```python
from build123d import *

# Parameters (mm, degrees)
SKETCH_1_W          = 35.997280892
SKETCH_1_H          = 36.282611102
SKETCH_1_W_2        = 35
SKETCH_1_H_2        = 32
EXTRUDE_1_DEPTH     = 65
SKETCH_1_3_W        = 35.997280892
SKETCH_1_3_H        = 36.282611102
SKETCH_1_3_W_2      = 35
SKETCH_1_3_H_2      = 32
EXTRUDE_2_DEPTH     = 2
SKETCH_2_R          = 1
CUT_EXTRUDE_1_DEPTH = 74.759079051
SKETCH_3_R          = 2
CUT_EXTRUDE_2_DEPTH = 1
EXTRUDE_3_DEPTH     = 4.5
EXTRUDE_4_DEPTH     = 30


with BuildPart() as part:
    # Sketch 1 → Extrude 1 (new body)
    # profile 1 of 5: a face of its own
    with BuildSketch(Plane(origin=(0, 0, 0), x_dir=(1, 0, 0), z_dir=(0, 1, 0))):
        Polygon((-14.328756252, 21.811189745), (14.328756252, 21.811189745), (17.998640446, 18.141305551), (-17.998640446, 18.141305551), align=None)
    # profile 2 of 5: a face of its own
    with BuildSketch(Plane(origin=(0, 0, 0), x_dir=(1, 0, 0), z_dir=(0, 1, 0))):
        Rectangle(SKETCH_1_W, SKETCH_1_H)
        Rectangle(SKETCH_1_W_2, SKETCH_1_H_2, mode=Mode.SUBTRACT)
    # profile 3 of 5: a face of its own
    with BuildSketch(Plane(origin=(0, 0, 0), x_dir=(1, 0, 0), z_dir=(0, 1, 0))):
        Polygon((-21.809945997, -14.33), (-21.809945997, 14.33), (-17.998640446, 18.141305551), (-17.998640446, -18.141305551), align=None)
    # profile 4 of 5: a face of its own
    with BuildSketch(Plane(origin=(0, 0, 0), x_dir=(1, 0, 0), z_dir=(0, 1, 0))):
        Polygon((14.328756252, -21.811189745), (-14.328756252, -21.811189745), (-17.998640446, -18.141305551), (17.998640446, -18.141305551), align=None)
    # profile 5 of 5: a face of its own
    with BuildSketch(Plane(origin=(0, 0, 0), x_dir=(1, 0, 0), z_dir=(0, 1, 0))):
        Polygon((21.809945997, 14.33), (21.809945997, -14.33), (17.998640446, -18.141305551), (17.998640446, 18.141305551), align=None)
    extrude(amount=EXTRUDE_1_DEPTH)

    # Sketch 1_3 → Extrude 2 (add)
    # profile 1 of 6: a face of its own
    with BuildSketch(Plane(origin=(0, 0, 0), x_dir=(1, 0, 0), z_dir=(0, 1, 0))):
        Polygon((-21.809945997, -14.33), (-21.809945997, 14.33), (-17.998640446, 18.141305551), (-17.998640446, -18.141305551), align=None)
    # profile 2 of 6: a face of its own
    with BuildSketch(Plane(origin=(0, 0, 0), x_dir=(1, 0, 0), z_dir=(0, 1, 0))):
        Rectangle(SKETCH_1_3_W, SKETCH_1_3_H)
        Rectangle(SKETCH_1_3_W_2, SKETCH_1_3_H_2, mode=Mode.SUBTRACT)
    # profile 3 of 6: a face of its own
    with BuildSketch(Plane(origin=(0, 0, 0), x_dir=(1, 0, 0), z_dir=(0, 1, 0))):
        Rectangle(SKETCH_1_3_W_2, SKETCH_1_3_H_2)
    # profile 4 of 6: a face of its own
    with BuildSketch(Plane(origin=(0, 0, 0), x_dir=(1, 0, 0), z_dir=(0, 1, 0))):
        Polygon((-14.328756252, 21.811189745), (14.328756252, 21.811189745), (17.998640446, 18.141305551), (-17.998640446, 18.141305551), align=None)
    # profile 5 of 6: a face of its own
    with BuildSketch(Plane(origin=(0, 0, 0), x_dir=(1, 0, 0), z_dir=(0, 1, 0))):
        Polygon((21.809945997, 14.33), (21.809945997, -14.33), (17.998640446, -18.141305551), (17.998640446, 18.141305551), align=None)
    # profile 6 of 6: a face of its own
    with BuildSketch(Plane(origin=(0, 0, 0), x_dir=(1, 0, 0), z_dir=(0, 1, 0))):
        Polygon((14.328756252, -21.811189745), (-14.328756252, -21.811189745), (-17.998640446, -18.141305551), (17.998640446, -18.141305551), align=None)
    extrude(amount=-EXTRUDE_2_DEPTH)

    # Sketch 2 → Cut-Extrude 1 (cut, through all)
    with BuildSketch(Plane.XZ.offset(2)):
        with Locations(Location((-3.809945997, 8, 0), (0, 0, 270))):
            Circle(SKETCH_2_R)
        with Locations(Location((-3.809945997, -8, 0), (0, 0, 270))):
            Circle(SKETCH_2_R)
    extrude(amount=-CUT_EXTRUDE_1_DEPTH, mode=Mode.SUBTRACT)

    # Sketch 3 → Cut-Extrude 2 (cut)
    with BuildSketch(Plane(origin=(0, 0, 0), x_dir=(1, 0, 0), z_dir=(0, 1, 0))):
        with Locations(Location((-3.809945997, 8, 0), (0, 0, 270))):
            Circle(SKETCH_3_R)
        with Locations(Location((-3.809945997, -8, 0), (0, 0, 270))):
            Circle(SKETCH_3_R)
    extrude(amount=-CUT_EXTRUDE_2_DEPTH, mode=Mode.SUBTRACT)

    # Sketch 4 → Extrude 3 (add)
    with BuildSketch(Plane.XZ.offset(2)):
        Polygon((-14.328756252, 21.811189745), (-19.27850372, 16.861442277), (-17.864290158, 15.447228714), (-12.91454269, 20.396976183), align=None)
        Polygon((19.27850372, 16.861442277), (14.328756252, 21.811189745), (12.91454269, 20.396976183), (17.864290158, 15.447228714), align=None)
        Polygon((12.91454269, -20.396976183), (14.328756252, -21.811189745), (19.27850372, -16.861442277), (17.864290158, -15.447228714), align=None)
        Polygon((-17.864290158, -15.447228714), (-19.27850372, -16.861442277), (-14.328756252, -21.811189745), (-12.91454269, -20.396976183), align=None)
    extrude(amount=EXTRUDE_3_DEPTH)

    # Sketch 5 → Extrude 4 (add)
    with BuildSketch(Plane.XZ.offset(2)):
        with BuildLine():
            ThreePointArc((8.828756252, 21.811189745), (5.891921221, 22.764586231), (4.075073469, 25.261189745))
            Line((4.075073469, 25.261189745), (4.075073469, 21.811189745))
            Line((4.075073469, 21.811189745), (8.828756252, 21.811189745))
        make_face()
        with BuildLine():
            ThreePointArc((13.582439035, 25.261189745), (11.765591283, 22.764586231), (8.828756252, 21.811189745))
            Line((8.828756252, 21.811189745), (13.582439035, 21.811189745))
            Line((13.582439035, 21.811189745), (13.582439035, 25.261189745))
        make_face()
    extrude(amount=-EXTRUDE_4_DEPTH)


solid = part.part
```
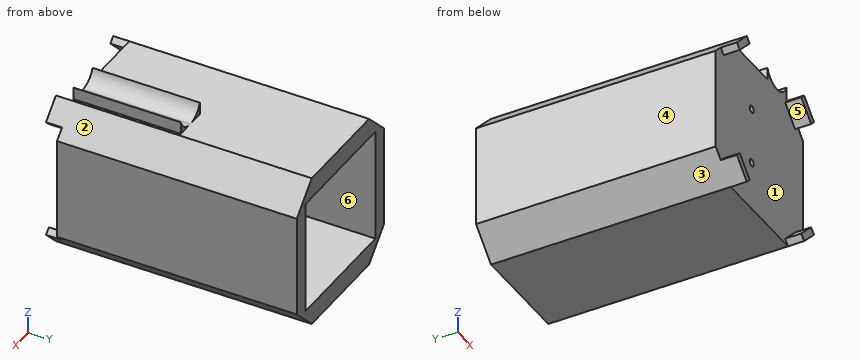
Work out the finished part from the listing and answer in its coordinate system (mm). Face numbers are marked on the shaded views. A direction names the side the tool comes from. Round coordinates to 2 decimals unless told otherwise and drop trailing zeros. Write each loop counter-clockwise with the first axis right and the second up, starting at its lowest first coordinate (ties: lowest second). Pieces come first, ordered by that corner, then holes. Notation, with made-up numbers: (24, 65.5) - (75, 65.5) arc R19 ccw to (75, 90.5) - close; hole circle Ø9 at (59, 61.5). An arc over 180 degrees is marked (long way). Return JSON: item names as keys, results as strings. Group by question number.
Q1. The mould has two halves that part along X. Classify the marked faces 1, 2 and 3: released by +X, released by -X, zero draft, split by the parting line, or undercut.
Q2. The part is cut by section D-D on x = 11. Write down the section's boundary in (y, z).
Q3. The part is cut by section A-A on z = 8. Write down the section's boundary in (x, y).
Q4. The part is cut by section C-C on z = 2. Write down the section's boundary in (x, y), then the cut area to 3 significant figures.
Q5. The part is cut by section B-B on y = 2. Write down the section's boundary in (x, z), then the cut area to 3 significant figures.
Q6. Each of these flat-tipped pins is pushed along its axis until it touches: pin 1 Ø1 at (y, z) = (8.5, 16) entering from +X; pin 2 Ø3 at (x, z) = (-4, -8) entering from +Y; pin 3 Ø13 at (x, z) = (-8, 5) entering from -Y. Where does it stop, or does it pass through?
Q7. Find the intervals of material crossed by L1, parallel to X at y = 36.5, z = -3.5; L2, parallel to Z at x = -0.5, y = 61; L3, parallel to X at y = -0.55, z = -8, in increasing order.
Q8. For the marked faces 4, 5 and 6, determine the directions among +Z, -Z, +X, -X, +Y, -Y from which every point of the face is accessible in a straight line to the end or side of a thin tool.
Solved:
{
 "1": {"face 1": "undercut", "face 2": "released by +X", "face 3": "released by -X"},
 "2": {"outline": "(-2, -21.81) - (65, -21.81) - (65, -16) - (0, -16) - (0, 16) - (65, 16) - (65, 21.81) - (28, 21.81) - (28, 22.31) - (-2, 22.31) - close"},
 "3": {"outline": "(-21.81, -2) - (-4.81, -2) - (-4.81, -1) - (-5.81, -1) - (-5.81, 0) - (-17.5, 0) - (-17.5, 65) - (-21.81, 65) - close; (-2.81, -2) - (21.81, -2) - (21.81, 65) - (17.5, 65) - (17.5, 0) - (-1.81, 0) - (-1.81, -1) - (-2.81, -1) - close"},
 "4": {"outline": "(-21.81, -2) - (21.81, -2) - (21.81, 65) - (17.5, 65) - (17.5, 0) - (-17.5, 0) - (-17.5, 65) - (-21.81, 65) - close", "area": "648 mm²"},
 "5": {"outline": "(-21.81, -14.33) - (-14.33, -21.81) - (14.33, -21.81) - (21.81, -14.33) - (21.81, 14.33) - (14.33, 21.81) - (13.58, 21.81) - (13.58, 25.26) arc R5 cw to (4.08, 25.26) - (4.08, 21.81) - (-14.33, 21.81) - (-21.81, 14.33) - close; hole (-17.5, -16) - (17.5, -16) - (17.5, 16) - (-17.5, 16) - close", "area": "680 mm²"},
 "6": {"pin 1": "x = 20.64", "pin 2": "y = -1", "pin 3": "y = -2"},
 "7": {"L1": "-21.81 to -17.5, 17.5 to 21.81", "L2": "-21.81 to -16, 16 to 21.81", "L3": "-21.81 to -5.81, -1.81 to 21.81"},
 "8": {"face 4": "+Z, -Z, -X, +Y, -Y", "face 5": "-Y", "face 6": "+Y"}
}
